Can you work these out from the model? Positions are in its coordinate system, mm. Face numbers are marked on the shaded views. A direction names the side the tool comes from. Coordinates: 2 decimals unless noted, no trailing zeros. Order: outer loops, then holes, each group sorted by start corner. A loop starts at its lowest first (then second) coordinate and runs counter-clockwise, first axis right, second up. Notation, with made-up numbers: (16, 84.5) -> (40, 84.5) arc R30 ccw to (40, 117.5) -> close; hole circle Ø10 at (34.5, 36). An arc over 180 degrees is marked (long way). Write item = value, one per line.
```python
from build123d import *

# Parameters (mm, degrees)
SKETCH_1_R               = 4
SKETCH_1_R_2             = 5.5
EXTRUDE_1_DEPTH          = 60
FILLET_1_R               = 10
SKETCH_2_R               = 12.5
EXTRUDE_2_DEPTH          = 30
HOLE_WIZARD_G3_8_1_D     = 15.25
HOLE_WIZARD_G3_8_1_DEPTH = 10
HOLE_WIZARD_G3_8_1_TIP   = 4.58156222
EXTRUDE_3_DEPTH          = 8
FILLET_2_R               = 2
FILLET_3_R               = 2


with BuildPart() as part:
    # 草图1 → 凸台-拉伸1 (new body)
    with BuildSketch(Plane.XY):
        with BuildLine():
            Line((-6.5, 25), (-6.5, 20))
            Line((-6.5, 20), (-47, 20))
            Line((-47, 20), (-47, -20))
            Line((-47, -20), (-6.5, -20))
            Line((-6.5, -20), (-6.5, -22))
            ThreePointArc((-6.5, -22), (0, -28.5), (6.5, -22))
            Line((6.5, -22), (6.5, -20))
            Line((6.5, -20), (17, -20))
            Line((17, -20), (17, 20))
            Line((17, 20), (6.5, 20))
            Line((6.5, 20), (6.5, 25))
            ThreePointArc((6.5, 25), (0, 31.5), (-6.5, 25))
        make_face()
        with Locations((0, 25)):
            Circle(SKETCH_1_R, mode=Mode.SUBTRACT)
        with Locations((0, -22)):
            Circle(SKETCH_1_R, mode=Mode.SUBTRACT)
        Circle(SKETCH_1_R_2, mode=Mode.SUBTRACT)
    extrude(amount=EXTRUDE_1_DEPTH)

    # 圆角1
    fillet_1_edges = [part.edges().sort_by_distance(p)[0] for p in [
        (-47, 0, 60),
    ]]
    fillet(fillet_1_edges, radius=FILLET_1_R)

    # 草图2 → 凸台-拉伸2 (add)
    with BuildSketch(Plane.XY.offset(60)):
        Circle(SKETCH_2_R)
    extrude(amount=EXTRUDE_2_DEPTH)

    # G3/8 螺纹孔1
    with Locations(Plane(origin=(0, -20, 0), x_dir=(-1, 0, 0), z_dir=(0, -1, 0))):
        with Locations((33, -46)):
            Hole(HOLE_WIZARD_G3_8_1_D / 2, depth=HOLE_WIZARD_G3_8_1_DEPTH)
            with Locations((0, 0, -(HOLE_WIZARD_G3_8_1_DEPTH + HOLE_WIZARD_G3_8_1_TIP / 2))):  # 118° drill point
                Cone(0, HOLE_WIZARD_G3_8_1_D / 2, HOLE_WIZARD_G3_8_1_TIP, mode=Mode.SUBTRACT)

    # 草图6 → 凸台-拉伸3 (add)
    with BuildSketch(Plane.XY.offset(90)):
        Polygon((9.814954576, 0), (4.907477288, 8.5), (-4.907477288, 8.5), (-9.814954576, 0), (-4.907477288, -8.5), (4.907477288, -8.5), align=None)
    extrude(amount=EXTRUDE_3_DEPTH)

    # 圆角2
    fillet_2_edges = [part.edges().sort_by_distance(p)[0] for p in [
        (17, 20, 30),
        (17, -20, 30),
        (-12.5, 0, 90),
    ]]
    fillet(fillet_2_edges, radius=FILLET_2_R)

    # 圆角3
    fillet_3_edges = [part.edges().sort_by_distance(p)[0] for p in [
        (4.907477288, -8.5, 94),
        (9.814954576, 0, 94),
        (4.907477288, 8.5, 94),
        (-4.907477288, 8.5, 94),
        (-9.814954576, 0, 94),
        (-4.907477288, -8.5, 94),
    ]]
    fillet(fillet_3_edges, radius=FILLET_3_R)

    # 草图7 → 切除-旋转1 (revolve, cut)
    with BuildSketch(Plane(origin=(0, 0, 0), x_dir=(1, 0, 0), z_dir=(0, 1, 0))):
        Polygon((-9.505553499, -96.994446501), (-8.5, -98), (-9.505553499, -98), align=None)
    revolve(axis=Axis((0, 0, -9.70684158), (0, 0, 1)), mode=Mode.SUBTRACT)


solid = part.part
```
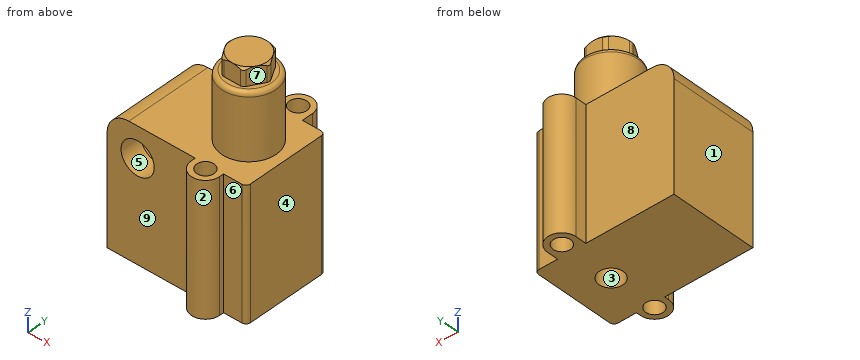
Item 1: I want a section at B-B, the plane z = 63. Please give me the cut outline in (x, y), plus the area to 3 significant figures.
A:
outline = circle Ø25 at (0, 0)
area = 491 mm2
Item 2: For the marked faces 5, 6, 7, 8 and 9, which set-ups out of +Z, -Z, +X, -X, +Y, -Y let a thin tool reach every point of the face, with its end or its side?
A:
face_5 = -Y
face_6 = +Z, -Z, +X, -Y
face_7 = +Z, +X, -Y
face_8 = +Z, -Z, -X, +Y
face_9 = +Z, -Z, -X, -Y
Item 3: If I drill on probe 1 along Y at (x, z) = (0, 34); probe 2 along Z at (x, y) = (-33, -13) (3 decimals); probe 3 along Z at (x, y) = (6, 22), over which ranges is the centre line in solid material (lowest first)?
A:
probe_1 = -28.5 to -26, -18 to -5.5, 5.5 to 21, 29 to 31.5
probe_2 = 0 to 38.375, 53.625 to 60
probe_3 = 0 to 60
Item 4: I want a section at A-A, the plane z = 36. Please give me the cut outline in (x, y), plus the area to 3 significant figures.
A:
outline = (-47, -20) -> (-6.5, -20) -> (-6.5, -22) arc R6.5 ccw to (6.5, -22) -> (6.5, -20) -> (15, -20) arc R2 ccw to (17, -18) -> (17, 18) arc R2 ccw to (15, 20) -> (6.5, 20) -> (6.5, 25) arc R6.5 ccw to (-6.5, 25) -> (-6.5, 20) -> (-47, 20) -> close; hole circle Ø11 at (0, 0); hole circle Ø8 at (0, -22); hole circle Ø8 at (0, 25)
area = 2,590 mm2
Item 5: If we mould it in two halves opening along X, with no side actions, what happens to the marked faces 1, 2, 3 and 4? For each: pulls with the +X half, pulls with the -X half, needs draft (parallel to the pull), parting line crosses it, or undercut.
A:
face_1 = pulls with the -X half
face_2 = parting line crosses it
face_3 = undercut
face_4 = pulls with the +X half
Item 6: I'm going to push flat-ended pins straight in: P1, Ø12, axis at x = 6.5, z = 71, coming from the -Y side; P2, Ø6, axis at x = -9.5, z = 69.5, coming from the -Y side; P3, Ø10, axis at x = -15, z = 31, coming from the +Y side. Where does each tip first touch, or does it pass through?
A:
P1 = -12.49
P2 = -10.68
P3 = 20
